```python
from build123d import *

# Parameters (mm, degrees)
F0_R     = 5.5000017
F1_DEPTH = 2.999994
F2_R     = 2.499995
F2_W     = 0.7533299053
F2_H     = 0.7162170781
F2_W_2   = 0.5293672881
F2_H_2   = 0.5760601295
F2_W_3   = 0.6473100061
F2_H_3   = 0.7012212299
F2_W_4   = 0.3967036741
F2_H_4   = 0.5668902525
F2_W_5   = 0.5837015153
F2_H_5   = 1.7340490769
F2_W_6   = 0.5672975831
F2_H_6   = 1.9103930295
F3_DEPTH = 0.0508


with BuildPart() as f1:
    # F0 (on Front) → F1 (new body)
    with BuildSketch(Plane.XZ):
        Circle(F0_R)
        Polygon((2.499995, -4.0000047), (-2.499995, -4.0000047), (-4.8093987903, 0), (-2.499995, 4.0000047), (2.499995, 4.0000047), (4.8093987903, 0), align=None, mode=Mode.SUBTRACT)
    extrude(amount=F1_DEPTH)

    # F2 (on Front) → F3 (join)
    with BuildSketch(Plane.XZ):
        Polygon((-3.3830750486, -2.5726628955), (-3.3830750486, -4.0979331759), (3.3830750486, -4.0979331759), (3.3830750486, -2.7493634261), (3.3830750486, -2.1733032967), (3.3830750486, 2.3381632997), (3.3830750486, 2.9050535522), (3.3830750486, 4.0979331759), (-3.3830750486, 4.0979331759), (-3.3830750486, 2.7106830385), (-3.3830750486, 2.0094618085), (-3.3830750486, -1.8564458175), align=None)
        Circle(F2_R, mode=Mode.SUBTRACT)
        with Locations((-3.7597400012, -2.2145543565)):
            Rectangle(F2_W, F2_H)
        with Locations((3.6477586926, -2.4613333614)):
            Rectangle(F2_W_2, F2_H_2)
        Polygon((-4.1364049539, -1.8564458175), (-3.3830750486, -1.8564458175), (-3.3830750486, 2.0094618085), (-4.0303850546, 2.0094618085), (-4.5122085367, 2.0094618085), (-4.5122085367, 0.8686301033), (-4.5122085367, -0.8654189736), (-4.5122085367, -1.8564458175), align=None)
        Polygon((3.3830750486, 2.3381632997), (3.3830750486, -2.1733032967), (3.9124423367, -2.1733032967), (4.4418096248, -2.1733032967), (4.4418096248, -0.8654189736), (4.4418096248, 1.0449740559), (4.4418096248, 2.3381632997), (3.7797787227, 2.3381632997), align=None)
        with Locations((-3.7067300516, 2.3600724235)):
            Rectangle(F2_W_3, F2_H_3)
        with Locations((3.5814268856, 2.621608426)):
            Rectangle(F2_W_4, F2_H_4)
        with Locations((-4.8040592943, 0.0016055649)):
            Rectangle(F2_W_5, F2_H_5)
        with Locations((4.7254584164, 0.0897775412)):
            Rectangle(F2_W_6, F2_H_6)
    extrude(amount=F3_DEPTH)


solid = f1.part
```
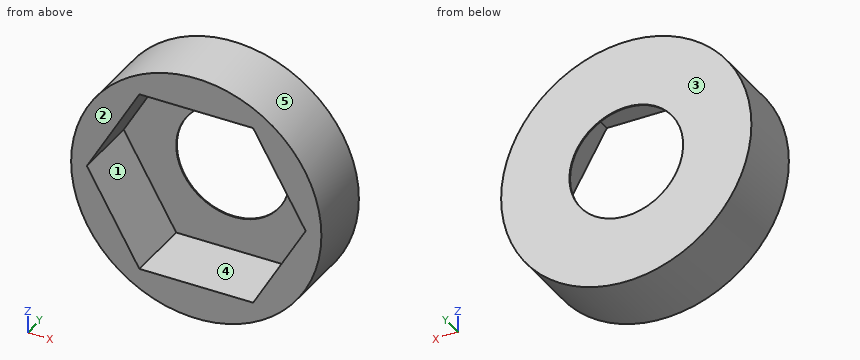
Check sheet for the modelled part. Datum: model origin and axes. Units: mm. Face numbers are marked on the shaded views. A direction names the side the tool comes from. Give positions to 0.01 mm unless a question says otherwise; leave off trailing zeros. Loops run counter-clockwise (first coordinate to the right, second up) from the corner with the lowest first, then second, coordinate; pieces in that order, holes last. Notation, with made-up numbers: M -19,-2.75 L 2,-2.75 A20 cw 2,21.25 Z; hole C 43,62 d4. An arc over 180 degrees is marked long. Answer in a Markdown table with one row per item.
1) Mould release check, pull along Z, two halves, no side actions. Record for the marked faces 3, 4 and 5: released by +Z, released by -Z, zero draft, split by the parting line, or undercut.
Solutions:
| item | result |
|---|---|
| face 3 | zero draft |
| face 4 | undercut |
| face 5 | split by the parting line |
2) Cross-section at A-A (x = 0). Enter the section's corners in (y, z).
Solutions:
| item | result |
|---|---|
| outline | M -3,-5.5 L 0,-5.5 L 0,-2.5 L -0.05,-2.5 L -0.05,-4 L -3,-4 Z; M -3,4 L -0.05,4 L -0.05,2.5 L 0,2.5 L 0,5.5 L -3,5.5 Z |
3) Thickness scan on line 1 (X direction, y = -2.75, z = -3); line 2 (Z direction, x = 0.5, y = -0.5); line 3 (Z direction, x = 1.25, y = -0.85). Record the ranges inside material, lowest first.
Solutions:
| item | result |
|---|---|
| line 1 | x = -4.61 to -3.08, 3.08 to 4.61 |
| line 2 | z = -5.48 to -4, 4 to 5.48 |
| line 3 | z = -5.36 to -4, 4 to 5.36 |
4) Cross-section at C-C (y = -0.35). Enter the section's corners in (x, z).
Solutions:
| item | result |
|---|---|
| outline | C 0,0 d11; hole M -4.81,0 L -2.5,-4 L 2.5,-4 L 4.81,0 L 2.5,4 L -2.5,4 Z |
5) Cross-section at D-D (x = 4.25). Enter the section's corners in (y, z).
Solutions:
| item | result |
|---|---|
| outline | M -3,-3.49 L 0,-3.49 L 0,3.49 L -3,3.49 L -3,0.97 L -0.05,0.97 L -0.05,-0.97 L -3,-0.97 Z |
6) Tool access check on the marked faces 1 and 2. Record the directions out of +Z, -Z, +X, -X, +Y, -Y that give a thin tool (end or side, any length) a straight path to the whole face; none if there is none.
Solutions:
| item | result |
|---|---|
| face 1 | -Y |
| face 2 | +Z, -Z, +X, -X, -Y |
7) Cross-section at B-B (z = 0.25). Enter the section's corners in (x, y), plus the area to 3 significant figures.
Solutions:
| item | result |
|---|---|
| outline | M -5.49,-3 L -4.67,-3 L -4.67,-0.05 L -2.49,-0.05 L -2.49,0 L -5.49,0 Z; M 2.49,-0.05 L 4.67,-0.05 L 4.67,-3 L 5.49,-3 L 5.49,0 L 2.49,0 Z |
| area | 5.20 mm^2 |
8) Depth check by flat-ended pin: pin 1 (0.9 mm diameter, centred on x = 1, y = -2, fed in from -Z); pin 2 (0.9 mm diameter, centred on x = 1, y = -1.5, fed in from +Z); pin 3 (5.5 mm diameter, centred on x = 0, z = 0, fed in from -Y); pin 4 (2.5 mm diameter, centred on x = -0.5, z = 0, fed in from -Y). Enter the tip coordinate at first touch or a pass-through.
Solutions:
| item | result |
|---|---|
| pin 1 | stops at z = -5.47 |
| pin 2 | stops at z = 5.47 |
| pin 3 | stops at y = -0.05 |
| pin 4 | passes through |
